```python
from build123d import *

# Parameters (mm, degrees)
BOSS_EXTRUDE2_DEPTH      = 5.3975
SKETCH2_W                = 19.05
SKETCH2_H                = 13.716
CUT_EXTRUDE1_DEPTH       = 107.104395791
SKETCH3_R                = 38.1
CUT_EXTRUDE2_DEPTH       = 107.104395791
FILLET1_R                = 6.35
SKETCH8_R                = 1.651
CUT_EXTRUDE7_DEPTH       = 75.692
SKETCH10_R               = 1.651
CUT_EXTRUDE9_DEPTH       = 97.79
SKETCH11_R               = 1.651
CUT_EXTRUDE10_DEPTH      = 150.876
SKETCH12_R               = 3.175
CUT_EXTRUDE11_DEPTH      = 103.378
CUT_EXTRUDE11_DEPTH_BACK = 48.768
SKETCH13_R               = 6.35
CUT_EXTRUDE12_DEPTH      = 26.416
SKETCH14_W               = 19.05
SKETCH14_H               = 13.716
CUT_EXTRUDE13_DEPTH      = 107.104395938
CUT_EXTRUDE14_DEPTH      = 107.104395938
FILLET2_R                = 2.54
FILLET3_R                = 2.54


with BuildPart() as part:
    # Sketch1 → Boss-Extrude2 (new body)
    with BuildSketch(Plane.XY):
        with BuildLine():
            ThreePointArc((-69.525975721, 27.94), (-74.93, 0), (-69.525975721, -27.94))
            ThreePointArc((-69.525975721, -27.94), (0, -74.93), (69.525975721, -27.94))
            ThreePointArc((69.525975721, -27.94), (73.56658977, -14.228906128), (74.93, 0))
            ThreePointArc((74.93, 0), (73.56658977, 14.228906128), (69.525975721, 27.94))
            ThreePointArc((69.525975721, 27.94), (0, 74.93), (-69.525975721, 27.94))
        make_face()
        Polygon((-67.493975721, 27.686), (-66.223975721, 27.686), (-56.063975721, 27.686), (-56.063975721, -27.686), (-66.223975721, -27.686), (-67.493975721, -27.686), (-67.493975721, -26.416), (-67.493975721, 26.416), align=None, mode=Mode.SUBTRACT)
        Polygon((67.493975721, 27.686), (67.493975721, 26.416), (67.493975721, -26.416), (67.493975721, -27.686), (66.223975721, -27.686), (56.063975721, -27.686), (56.063975721, 27.686), (66.223975721, 27.686), align=None, mode=Mode.SUBTRACT)
    extrude(amount=BOSS_EXTRUDE2_DEPTH)

    # Sketch2 → Cut-Extrude1 (cut, through all)
    with BuildSketch(Plane.XY.offset(5.3975)):
        with Locations((0, 62.23)):
            Rectangle(SKETCH2_W, SKETCH2_H)
    extrude(amount=-CUT_EXTRUDE1_DEPTH, mode=Mode.SUBTRACT)

    # Sketch3 → Cut-Extrude2 (cut, through all)
    with BuildSketch(Plane.XY.offset(5.3975)):
        with Locations((0, -86.312058398)):
            Circle(SKETCH3_R)
    extrude(amount=-CUT_EXTRUDE2_DEPTH, mode=Mode.SUBTRACT)

    # Fillet1
    fillet1_edges = [part.edges().sort_by_distance(p)[0] for p in [
        (-33.000960548, -67.271401821, 2.69875),
        (33.000960548, -67.271401821, 2.69875),
    ]]
    fillet(fillet1_edges, radius=FILLET1_R)

    # Sketch8 → Cut-Extrude7 (cut)
    with BuildSketch(Plane(origin=(30.092005081, 4.08352975, -11.4935), x_dir=(-1, 0, 0), z_dir=(0, 0, -1))):
        with Locations(Location((63.757223581, 17.50647025, 0), (0, 0, 180))):
            Circle(SKETCH8_R)
        with Locations(Location((63.757223581, -25.67352975, 0), (0, 0, 180))):
            Circle(SKETCH8_R)
        with Locations(Location((-3.552776419, -25.67352975, 0), (0, 0, 180))):
            Circle(SKETCH8_R)
        with Locations(Location((-3.552776419, 17.50647025, 0), (0, 0, 180))):
            Circle(SKETCH8_R)
    extrude(amount=-CUT_EXTRUDE7_DEPTH, mode=Mode.SUBTRACT)

    # Sketch10 → Cut-Extrude9 (cut)
    with BuildSketch(Plane(origin=(30.092005081, 4.08352975, -41.529), x_dir=(-1, 0, 0), z_dir=(0, 0, -1))):
        with Locations(Location((4.154396091, -49.728759131, 0), (0, 0, 180))):
            Circle(SKETCH10_R)
        with Locations(Location((56.02961407, -49.728759131, 0), (0, 0, 180))):
            Circle(SKETCH10_R)
        with Locations(Location((4.154396091, 41.38247025, 0), (0, 0, 180))):
            Circle(SKETCH10_R)
        with Locations(Location((56.02961407, 41.38247025, 0), (0, 0, 180))):
            Circle(SKETCH10_R)
    extrude(amount=-CUT_EXTRUDE9_DEPTH, mode=Mode.SUBTRACT)

    # Sketch11 → Cut-Extrude10 (cut)
    with BuildSketch(Plane(origin=(30.092005081, 4.08352975, 5.3975), x_dir=(1, 0, 0), z_dir=(0, 0, 1))):
        with Locations((-101.395980802, -12.71952975)):
            Circle(SKETCH11_R)
        with Locations((-101.395980802, 4.55247025)):
            Circle(SKETCH11_R)
        with Locations((41.211970641, -12.71952975)):
            Circle(SKETCH11_R)
        with Locations((41.211970641, 4.55247025)):
            Circle(SKETCH11_R)
    extrude(amount=-CUT_EXTRUDE10_DEPTH, mode=Mode.SUBTRACT)

    # Sketch12 → Cut-Extrude11 (cut, two sides)
    with BuildSketch(Plane(origin=(30.092005081, 4.08352975, -5.3975), x_dir=(-1, 0, 0), z_dir=(0, 0, -1))) as cut_extrude11_sk:
        with Locations(Location((-16.897994919, 21.31647025, 0), (0, 0, 180))):
            Circle(SKETCH12_R)
        with Locations(Location((77.082005081, 21.31647025, 0), (0, 0, 180))):
            Circle(SKETCH12_R)
        with Locations(Location((30.092005081, 21.31647025, 0), (0, 0, 180))):
            Circle(SKETCH12_R)
        with Locations(Location((77.082005081, -29.48352975, 0), (0, 0, 180))):
            Circle(SKETCH12_R)
        with Locations(Location((30.092005081, -29.48352975, 0), (0, 0, 180))):
            Circle(SKETCH12_R)
        with Locations(Location((-16.897994919, -29.48352975, 0), (0, 0, 180))):
            Circle(SKETCH12_R)
    extrude(amount=CUT_EXTRUDE11_DEPTH, mode=Mode.SUBTRACT)
    extrude(cut_extrude11_sk.sketch, amount=-CUT_EXTRUDE11_DEPTH_BACK, mode=Mode.SUBTRACT)

    # Sketch13 → Cut-Extrude12 (cut)
    with BuildSketch(Plane(origin=(0, 0, 0), x_dir=(-1, 0, 0), z_dir=(0, 0, -1))):
        with Locations((46.99, 25.4)):
            Circle(SKETCH13_R)
        with Locations((0, 25.4)):
            Circle(SKETCH13_R)
        with Locations((-46.99, 25.4)):
            Circle(SKETCH13_R)
        with Locations((-46.99, -25.4)):
            Circle(SKETCH13_R)
        with Locations((0, -25.4)):
            Circle(SKETCH13_R)
        with Locations((46.99, -25.4)):
            Circle(SKETCH13_R)
    extrude(amount=-CUT_EXTRUDE12_DEPTH, mode=Mode.SUBTRACT)

    # Sketch14 → Cut-Extrude13 (cut, through all)
    with BuildSketch(Plane.XY.offset(5.3975)):
        with Locations((0, -39.116)):
            Rectangle(SKETCH14_W, SKETCH14_H)
    extrude(amount=-CUT_EXTRUDE13_DEPTH, mode=Mode.SUBTRACT)

    # Sketch15 → Cut-Extrude14 (cut, through all)
    with BuildSketch(Plane(origin=(0, 0, 0), x_dir=(-1, 0, 0), z_dir=(0, 0, -1))):
        with BuildLine():
            ThreePointArc((67.493975721, -27.686), (68.149254897, -26.031335187), (68.763975721, -24.361178085))
            Line((68.763975721, -24.361178085), (68.763975721, 24.361178085))
            ThreePointArc((68.763975721, 24.361178085), (68.149254897, 26.031335187), (67.493975721, 27.686))
            Line((67.493975721, 27.686), (67.493975721, -27.686))
        make_face()
        with BuildLine():
            ThreePointArc((-68.763975721, -24.361178085), (-68.149254897, -26.031335187), (-67.493975721, -27.686))
            Line((-67.493975721, -27.686), (-67.493975721, 27.686))
            ThreePointArc((-67.493975721, 27.686), (-68.149254897, 26.031335187), (-68.763975721, 24.361178085))
            Line((-68.763975721, 24.361178085), (-68.763975721, -24.361178085))
        make_face()
    extrude(amount=-CUT_EXTRUDE14_DEPTH, mode=Mode.SUBTRACT)

    # Fillet2
    fillet2_edges = [part.edges().sort_by_distance(p)[0] for p in [
        (-67.493975721, 27.686, 2.69875),
        (-67.493975721, -27.686, 2.69875),
        (-68.763975721, 24.361178085, 2.69875),
        (-68.763975721, -24.361178085, 2.69875),
    ]]
    fillet(fillet2_edges, radius=FILLET2_R)

    # Fillet3
    fillet3_edges = [part.edges().sort_by_distance(p)[0] for p in [
        (67.493975721, -27.686, 2.69875),
        (67.493975721, 27.686, 2.69875),
        (68.763975721, -24.361178085, 2.69875),
        (68.763975721, 24.361178085, 2.69875),
    ]]
    fillet(fillet3_edges, radius=FILLET3_R)


solid = part.part
```
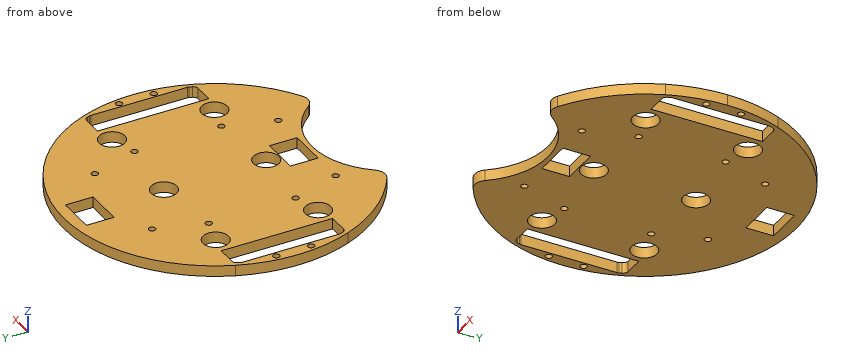
CAD build for the part. Positions are in the model's coordinates, mm. Round coordinates to 2 decimals unless told otherwise and drop trailing zeros. Write each loop counter-clockwise with the first axis right and the second up, starting at its lowest first coordinate (ties: lowest second). Pieces come first, ordered by that corner, then holes. Notation, with made-up numbers: (44.5, -21) -> (51.5, -21) arc R31 ccw to (51.5, 3) -> close; hole circle Ø9 at (81.5, 39.25). An arc over 180 degrees is marked (long way). Answer in a Markdown table with one row per item. Add a question column.
Item 1: Saw through at D-D, the plane y = -55. Write the cut outline in (x, z), then the cut area to 3 significant figures.
Item 2: Drill centre lines: line 1 (X direction, y = -2, z = 3.95); line 2 (Y direction, x = 46.99, z = 3.1); line 3 (Y direction, x = -50, z = 2.45). Where is each one in solid material? Low to high. Write a range as from..to.
Item 3: Saw through at C-C, the plane y = 21.59. Count the separate pieces of the cut face and the enclosed holes in it, then the cut area to 3 significant figures.
Item 4: Saw through at A-A, the plane x = 0. Write the cut outline in (y, z), then the cut area to 3 significant figures.
Item 5: Drop flat-ended pins along their axis: pin 1 Ø2 at (y, z) = (46.5, 2.5) entering from +X; pin 2 Ø2.5 at (x, y) = (25.94, -45.65) entering from -Z; pin 3 Ø2 at (y, z) = (-4, 2) entering from +X; pin 4 Ø1.5 at (y, z) = (58, 3) entering from -X. Give the stop position or say it passes through.
Item 6: Saw through at B-B, the plane x = -50. Write the cut outline in (y, z), then the cut area to 3 significant figures.
Findings below:
| question | item | result |
|---|---|---|
| 1 | outline | (-50.89, 0) -> (-21.71, 0) -> (-21.71, 5.4) -> (-50.89, 5.4) -> close; (21.71, 0) -> (50.89, 0) -> (50.89, 5.4) -> (21.71, 5.4) -> close |
| 1 | area | 315 mm^2 |
| 2 | line 1 | x = -74.9..-68.76, -56.06..56.06, 68.76..74.9 |
| 2 | line 2 | y = -58.36..-31.75, -19.05..19.05, 31.75..58.36 |
| 2 | line 3 | y = -55.81..-30.99, -19.81..19.81, 30.99..55.81 |
| 3 | separate pieces | 8 |
| 3 | enclosed holes | 0 |
| 3 | area | 437 mm^2 |
| 4 | outline | (-48.21, 0) -> (-45.97, 0) -> (-45.97, 5.4) -> (-48.21, 5.4) -> close; (-32.26, 0) -> (-31.75, 0) -> (-31.75, 5.4) -> (-32.26, 5.4) -> close; (-19.05, 0) -> (19.05, 0) -> (19.05, 5.4) -> (-19.05, 5.4) -> close; (31.75, 0) -> (55.37, 0) -> (55.37, 5.4) -> (31.75, 5.4) -> close; (69.09, 0) -> (74.93, 0) -> (74.93, 5.4) -> (69.09, 5.4) -> close |
| 4 | area | 379 mm^2 |
| 5 | pin 1 | stops at x = 59.53 |
| 5 | pin 2 | passes through |
| 5 | pin 3 | stops at x = 74.87 |
| 5 | pin 4 | stops at x = -48.34 |
| 6 | outline | (-55.81, 0) -> (-30.99, 0) -> (-30.99, 5.4) -> (-55.81, 5.4) -> close; (-19.81, 0) -> (19.81, 0) -> (19.81, 5.4) -> (-19.81, 5.4) -> close; (30.99, 0) -> (55.81, 0) -> (55.81, 5.4) -> (30.99, 5.4) -> close |
| 6 | area | 482 mm^2 |
